Check sheet for the modelled part. Datum: model origin and axes. Units: mm. A direction names the side the tool comes from. Round coordinates to 2 decimals unless told otherwise and drop trailing zeros. Order: outer loops, then holes, each group sorted by start corner. A loop starts at its lowest first (then second) coordinate and runs counter-clockwise, first axis right, second up.
(1) Tool access check on faces 1 (the flat face through (36.4, -2, 5)), 2 (the flat face through (48.4, 0, 5)), 3 (the flat face through (-30.4, -2, 5)). Record the directions out of +Z, -Z, +X, -X, +Y, -Y that give a thin tool (end or side, any length) a straight path to the whole face; none if there is none.
(2) Mould release check, pull along Z, two halves, no side actions. Record for faces 4 (the flat face through (-1, -1, 0)), 5 (the cylindrical face through (-42.07, -0.01, 5.69)), 6 (the flat face through (-48.4, 0, 5)), 7 (the cylindrical face through (44.41, -0.01, 6.11)): released by +Z, released by -Z, zero draft, split by the parting line, or undercut.
(3) Thickness scan on probe 1 along X at (y, z) = (-0.5, 5); probe 2 along Z at (x, y) = (-43.4, -0.2); probe 3 along X at (y, z) = (-0.15, 4.5). Record the ranges inside material, lowest first.
(4) Sectioned sample at B-B, the plane x = -43.4. Enter the section's corners in (y, z), and give its area (3 significant figures).
(5) Depth check by flat-ended pin: pin 1 (2.5 mm diameter, centred on x = -43.4, z = 5, fed in from -Y); pin 2 (1.6 mm diameter, centred on y = -2, z = 2.5, fed in from -X); pin 3 (0.6 mm diameter, centred on y = -2, z = 4.5, fed in from +X). Enter the tip coordinate at first touch or a pass-through.
(6) Sectioned sample at A-A, the plane z = 5. Enter the section's corners in (x, y).
(7) Sectioned sample at C-C, the plane z = 1. Enter the section's corners in (x, y).
```python
from build123d import *

# Parameters (mm, degrees)
CROQUIS2_W              = 96.8
CROQUIS2_H              = 2
SALIENTE_EXTRUIR2_DEPTH = 10
CROQUIS3_W              = 66.8
CROQUIS3_H              = 10
SALIENTE_EXTRUIR3_DEPTH = 2
CROQUIS5_R              = 1.5
CORTAR_EXTRUIR1_DEPTH   = 2


with BuildPart() as part:
    # Croquis2 → Saliente-Extruir2 (new body)
    with BuildSketch(Plane.XY):
        Rectangle(CROQUIS2_W, CROQUIS2_H)
    extrude(amount=SALIENTE_EXTRUIR2_DEPTH)

    # Croquis3 → Saliente-Extruir3 (add)
    with BuildSketch(Plane.XZ.offset(1)):
        with Locations((3, 5)):
            Rectangle(CROQUIS3_W, CROQUIS3_H)
    extrude(amount=SALIENTE_EXTRUIR3_DEPTH)

    # Croquis5 → Cortar-Extruir1 (cut)
    with BuildSketch(Plane.XZ.offset(1)):
        with Locations(Location((43.4, 5, 0), (0, 0, 270))):
            Circle(CROQUIS5_R)
        with Locations(Location((-43.4, 5, 0), (0, 0, 90))):
            Circle(CROQUIS5_R)
    extrude(amount=-CORTAR_EXTRUIR1_DEPTH, mode=Mode.SUBTRACT)


solid = part.part
```
Derived:
1. face 1: +Z, -Z, +X, -Y
1. face 2: +Z, -Z, +X, +Y, -Y
1. face 3: +Z, -Z, -X, -Y
2. face 4: released by -Z
2. face 5: undercut
2. face 6: zero draft
2. face 7: undercut
3. probe 1: x = -48.4 to -44.9, -41.9 to 41.9, 44.9 to 48.4
3. probe 2: z = 0 to 3.5, 6.5 to 10
3. probe 3: x = -48.4 to -44.81, -41.99 to 41.99, 44.81 to 48.4
4. outline: (-1, 0) - (1, 0) - (1, 3.5) - (-1, 3.5) - close; (-1, 6.5) - (1, 6.5) - (1, 10) - (-1, 10) - close
4. area: 14.0 mm2
5. pin 1: passes through
5. pin 2: stops at x = -30.4
5. pin 3: stops at x = 36.4
6. outline: (-48.4, -1) - (-44.9, -1) - (-44.9, 1) - (-48.4, 1) - close; (-41.9, -1) - (-30.4, -1) - (-30.4, -3) - (36.4, -3) - (36.4, -1) - (41.9, -1) - (41.9, 1) - (-41.9, 1) - close; (44.9, -1) - (48.4, -1) - (48.4, 1) - (44.9, 1) - close
7. outline: (-48.4, -1) - (-30.4, -1) - (-30.4, -3) - (36.4, -3) - (36.4, -1) - (48.4, -1) - (48.4, 1) - (-48.4, 1) - close
